from build123d import *

# Parameters (mm, degrees)
ESBO_O1_W                = 250
ESBO_O1_H                = 250
ESBO_O1_R                = 2
RESSALTO_EXTRUS_O1_DEPTH = 3
ESBO_O2_W                = 16.471941672
ESBO_O2_H                = 247.6
ESBO_O2_R                = 2
RESSALTO_EXTRUS_O2_DEPTH = 17
RESSALTO_EXTRUS_O3_DEPTH = 22


with BuildPart() as part:
    # Esbo_o1 → Ressalto-extrus_o1 (new body)
    with BuildSketch(Plane(origin=(0, 0, 0), x_dir=(1, 0, 0), z_dir=(0, 1, 0))):
        Rectangle(ESBO_O1_W, ESBO_O1_H)
        with Locations((-115, 115)):
            Circle(ESBO_O1_R, mode=Mode.SUBTRACT)
        with Locations((115, 115)):
            Circle(ESBO_O1_R, mode=Mode.SUBTRACT)
        with Locations((-115, -115)):
            Circle(ESBO_O1_R, mode=Mode.SUBTRACT)
        with Locations((115, -115)):
            Circle(ESBO_O1_R, mode=Mode.SUBTRACT)
    extrude(amount=RESSALTO_EXTRUS_O1_DEPTH)

    # Esbo_o2 → Ressalto-extrus_o2 (add)
    with BuildSketch(Plane(origin=(0, 3, 0), x_dir=(1, 0, 0), z_dir=(0, 1, 0))):
        with Locations((-116.764029164, 0)):
            Rectangle(ESBO_O2_W, ESBO_O2_H)
        with Locations((-115, -115)):
            Circle(ESBO_O2_R, mode=Mode.SUBTRACT)
        with Locations((-115, 115)):
            Circle(ESBO_O2_R, mode=Mode.SUBTRACT)
        with Locations((116.764029164, 0)):
            Rectangle(ESBO_O2_W, ESBO_O2_H)
        with Locations((115, -115)):
            Circle(ESBO_O2_R, mode=Mode.SUBTRACT)
        with Locations((115, 115)):
            Circle(ESBO_O2_R, mode=Mode.SUBTRACT)
    extrude(amount=RESSALTO_EXTRUS_O2_DEPTH)

    # Esbo_o2_5 → Ressalto-extrus_o3 (add)
    with BuildSketch(Plane(origin=(0, 3, 0), x_dir=(1, 0, 0), z_dir=(0, 1, 0))):
        Polygon((-125, 123.8), (-108.528058328, 123.8), (108.528058328, 123.8), (125, 123.8), (125, 125), (-125, 125), align=None)
        Polygon((108.528058328, -123.8), (-108.528058328, -123.8), (-125, -123.8), (-125, -125), (125, -125), (125, -123.8), align=None)
    extrude(amount=RESSALTO_EXTRUS_O3_DEPTH)


solid = part.part
Input: part model. Units: mm. Frame: model coordinates. A direction names the side the tool comes from. Round coordinates to 2 decimals unless told otherwise and drop trailing zeros. Order: outer loops, then holes, each group sorted by start corner. A loop starts at its lowest first (then second) coordinate and runs counter-clockwise, first axis right, second up. Notation, with made-up numbers: (45.25, 16.5) - (60.25, 16.5) arc R29 ccw to (60.25, 49.5) - close; hole circle Ø11 at (58.25, 33.5). An arc over 180 degrees is marked (long way). Answer as a JSON object with one key per item and string values. Group by question number.
(1) Cut plane C-C (x = 17.5). Return loops of the section in (y, z), then the cut area to 3 significant figures.
(2) Pin query (flat end, axial travel): P1, Ø1, axis at x = 31.5, z = 27, coming from the +Y side; P2, Ø3, axis at x = -115, z = 115, coming from the -Y side; P3, Ø5, axis at x = 116.5, z = -51.5, coming from the +Y side. Return the tip coordinate at first contact, or that it passes through.
(3) Reachability of faces 1 (the face through (-117, 20, -2)), 2 (the face through (108.528, 11, 2)), 3 (the face through (-2, 12, 125)) from +Z, -Z, +X, -X, +Y, -Y: full face, straight path, thin tool, end or side. Return the list, or none.
(4) Material intervals for probe 1 along Z at (x, y) = (-115, 13); probe 2 along X at (y, z) = (4.75, 115); probe 3 along Z at (x, y) = (2.5, 8.5), sorted ascending. Write a range as from..to.
(5) Cut plane B-B (z = 13). Return loops of the section in (x, y).
(6) Cut plane A-A (y = 11). Return loops of the section in (x, z).
Here are the results:
{
 "1": {"outline": "(0, -125) - (25, -125) - (25, -123.8) - (3, -123.8) - (3, 123.8) - (25, 123.8) - (25, 125) - (0, 125) - close", "area": "803 mm^2"},
 "2": {"P1": "stops at y = 3", "P2": "passes through", "P3": "stops at y = 20"},
 "3": {"face 1": "+X, -X, +Y", "face 2": "+Y", "face 3": "+Z, +X, -X, +Y, -Y"},
 "4": {"probe 1": "z = -125..-117, -113..113, 117..125", "probe 2": "x = -125..-117, -113..-108.53, 108.53..113, 117..125", "probe 3": "z = -125..-123.8, 123.8..125"},
 "5": {"outline": "(-125, 0) - (125, 0) - (125, 20) - (108.53, 20) - (108.53, 3) - (-108.53, 3) - (-108.53, 20) - (-125, 20) - close"},
 "6": {"outline": "(-125, -125) - (125, -125) - (125, 125) - (-125, 125) - close; hole circle Ø4 at (-115, -115); hole circle Ø4 at (-115, 115); hole (-108.53, -123.8) - (108.53, -123.8) - (108.53, 123.8) - (-108.53, 123.8) - close; hole circle Ø4 at (115, -115); hole circle Ø4 at (115, 115)"}
}
